from build123d import *

# Parameters (mm, degrees)
SKETCH1_W               = 150
SKETCH1_H               = 50
BOSS_EXTRUDE1_DEPTH     = 3
CUT_EXTRUDE1_DEPTH      = 80.113842025
CUT_EXTRUDE1_DEPTH_BACK = 80.113842025
SKETCH2_R               = 1.5
SKETCH3_R               = 5
CUT_EXTRUDE2_DEPTH      = 80.113842025


with BuildPart() as part:
    # Sketch1 → Boss-Extrude1 (new body)
    with BuildSketch(Plane(origin=(0, 0, 0), x_dir=(1, 0, 0), z_dir=(0, 1, 0))):
        Rectangle(SKETCH1_W, SKETCH1_H)
    extrude(amount=BOSS_EXTRUDE1_DEPTH)

    # Sketch2 → Cut-Extrude1 (cut, two sides: drawn at the far end of the back side and taken through both)
    with BuildSketch(Plane(origin=(0, 3, 0), x_dir=(1, 0, 0), z_dir=(0, 1, 0)).offset(-CUT_EXTRUDE1_DEPTH_BACK)):
        with Locations(Location((-55, 3.75, 0), (0, 0, 270))):
            Circle(SKETCH2_R)
        with Locations(Location((-55, -3.75, 0), (0, 0, 90))):
            Circle(SKETCH2_R)
        with Locations(Location((-25, -3.75, 0), (0, 0, 270))):
            Circle(SKETCH2_R)
        with Locations(Location((-25, 3.75, 0), (0, 0, 90))):
            Circle(SKETCH2_R)
    extrude(amount=CUT_EXTRUDE1_DEPTH + CUT_EXTRUDE1_DEPTH_BACK, mode=Mode.SUBTRACT)

    # Sketch3 → Cut-Extrude2 (cut, through all)
    with BuildSketch(Plane(origin=(0, 3, 0), x_dir=(1, 0, 0), z_dir=(0, 1, 0))):
        with Locations(Location((32, 0, 0), (0, 0, 270))):
            Circle(SKETCH3_R)
    extrude(amount=-CUT_EXTRUDE2_DEPTH, mode=Mode.SUBTRACT)


solid = part.part
Geometry check sheet. Reference: the model listing, model coordinates, mm. Round coordinates to 2 decimals unless told otherwise and drop trailing zeros. Order: outer loops, then holes, each group sorted by start corner. A loop starts at its lowest first (then second) coordinate and runs counter-clockwise, first axis right, second up. Notation, with made-up numbers: (68.25, 83.25) - (98.25, 83.25) arc R21 ccw to (98.25, 122.25) - close; hole circle Ø1 at (-35.5, 66.25). An arc over 180 degrees is marked (long way). One line per question, with ' | ' between items. Start each with the question number.
(1) Sectioned sample at A-A on z = 0. Record the cut outline in (x, y), and give its area (3 significant figures).
(2) Sectioned sample at C-C on x = -25. Record the cut outline in (y, z), and give its area (3 significant figures).
(3) Depth check by flat-ended pin: pin 1 Ø6 at (x, z) = (-10, -2.5) entering from -Y. Enter the tip coordinate at first touch or a pass-through.
(4) Release check for a two-part mould opening along Z. For faces 1 (the cylindrical face through (-23.735, 1.479, 4.556)), 2 (the flat face through (-1, 1, 25)), 3 (the flat face through (-1, 1, -25)), 4 (the flat face through (-75, 1, 0)) record: released by +Z, released by -Z, zero draft, split by the parting line, or undercut.
(5) Sectioned sample at B-B on x = 32. Record the cut outline in (y, z).
(6) Thickness scan on L1, parallel to X at y = 1.2, z = -3.75; L2, parallel to X at y = 0.8, z = -2. Record the ranges inside material, lowest first. Write a range as [from, to].
Conclusion:
1) outline: (-75, 0) - (27, 0) - (27, 3) - (-75, 3) - close; (37, 0) - (75, 0) - (75, 3) - (37, 3) - close | area: 420 mm2
2) outline: (0, -25) - (3, -25) - (3, -5.25) - (0, -5.25) - close; (0, -2.25) - (3, -2.25) - (3, 2.25) - (0, 2.25) - close; (0, 5.25) - (3, 5.25) - (3, 25) - (0, 25) - close | area: 132 mm2
3) pin 1: stops at y = 0
4) face 1: undercut | face 2: released by +Z | face 3: released by -Z | face 4: zero draft
5) outline: (0, -25) - (3, -25) - (3, -5) - (0, -5) - close; (0, 5) - (3, 5) - (3, 25) - (0, 25) - close
6) L1: x = [-75, -56.5], [-53.5, -26.5], [-23.5, 28.69], [35.31, 75] | L2: x = [-75, 27.42], [36.58, 75]
